Source: CAD feature listing. Evaluate the final solid. Frame: model axes, mm. Face numbers are marked on the shaded views. Round coordinates to 2 decimals unless told otherwise and drop trailing zeros. Write each loop counter-clockwise with the first axis right and the second up, starting at its lowest first coordinate (ties: lowest second). Pieces come first, ordered by that corner, then holes.
from build123d import *

# Parameters (mm, degrees)
SKETCH1_R           = 2.5
BOSS_EXTRUDE2_DEPTH = 6
SKETCH2_W           = 140.18
SKETCH2_H           = 28.64
CUT_EXTRUDE1_DEPTH  = 3


with BuildPart() as part:
    # Sketch1 → Boss-Extrude2 (new body)
    with BuildSketch(Plane(origin=(0, 0, 0), x_dir=(1, 0, 0), z_dir=(0, 1, 0))):
        Polygon((-85.09, 17.32), (-82.09, 20.32), (82.09, 20.32), (85.09, 17.32), (85.09, -17.32), (82.09, -20.32), (-82.09, -20.32), (-85.09, -17.32), align=None)
        with Locations(Location((-76.7, 12.7, 0), (0, 0, 270))):
            Circle(SKETCH1_R, mode=Mode.SUBTRACT)
        with Locations(Location((-76.7, -12.7, 0), (0, 0, 270))):
            Circle(SKETCH1_R, mode=Mode.SUBTRACT)
        with Locations(Location((76.7, 12.7, 0), (0, 0, 270))):
            Circle(SKETCH1_R, mode=Mode.SUBTRACT)
        with Locations(Location((76.7, -12.7, 0), (0, 0, 270))):
            Circle(SKETCH1_R, mode=Mode.SUBTRACT)
    extrude(amount=BOSS_EXTRUDE2_DEPTH)

    # Sketch2 → Cut-Extrude1 (cut)
    with BuildSketch(Plane(origin=(0, 6, 0), x_dir=(1, 0, 0), z_dir=(0, 1, 0))):
        Rectangle(SKETCH2_W, SKETCH2_H)
    extrude(amount=-CUT_EXTRUDE1_DEPTH, mode=Mode.SUBTRACT)


solid = part.part
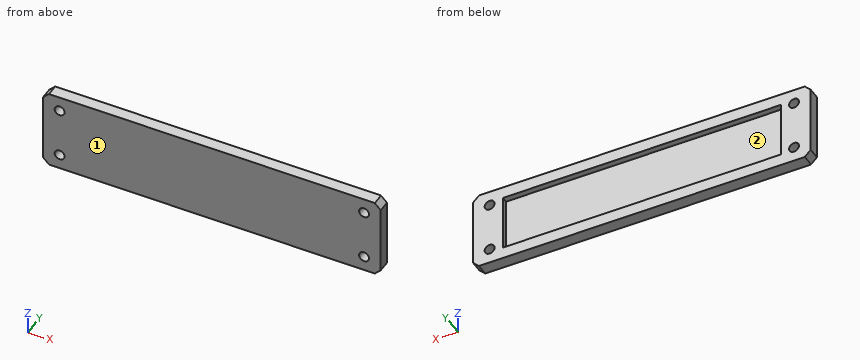
1) Contact query for a flat-ended pin moving along its axis: P1, Ø14.5, axis at x = -30, z = 2.5, coming from the +Y side. Output: stop coordinate, or through.
Taken from the geometry:
P1: stops at y = 3
2) Material intervals for line 1 (X direction, y = 3.2, z = -12.7); line 2 (X direction, y = 4.1, z = -10); line 3 (X direction, y = 2.85, z = 12.7), sorted ascending.
Taken from the geometry:
line 1: x = -85.09 to -79.2, -74.2 to -70.09, 70.09 to 74.2, 79.2 to 85.09
line 2: x = -85.09 to -70.09, 70.09 to 85.09
line 3: x = -85.09 to -79.2, -74.2 to 74.2, 79.2 to 85.09
3) Section query C-C on x = -76.7. Return the cut outline in (y, z), then the cut area to 3 significant figures.
Taken from the geometry:
outline: (0, -20.32) - (6, -20.32) - (6, -15.2) - (0, -15.2) - close; (0, -10.2) - (6, -10.2) - (6, 10.2) - (0, 10.2) - close; (0, 15.2) - (6, 15.2) - (6, 20.32) - (0, 20.32) - close
area: 184 mm2
4) Section query B-B on y = 4.75. Return the cut outline in (x, z), then the cut area to 3 significant figures.
Taken from the geometry:
outline: (-85.09, -17.32) - (-82.09, -20.32) - (82.09, -20.32) - (85.09, -17.32) - (85.09, 17.32) - (82.09, 20.32) - (-82.09, 20.32) - (-85.09, 17.32) - close; hole circle Ø5 at (-76.7, -12.7); hole circle Ø5 at (-76.7, 12.7); hole (-70.09, -14.32) - (70.09, -14.32) - (70.09, 14.32) - (-70.09, 14.32) - close; hole circle Ø5 at (76.7, -12.7); hole circle Ø5 at (76.7, 12.7)
area: 2,800 mm2
5) Section query D-D on z = 6.5. Return the cut outline in (x, y), then the cut area to 3 significant figures.
Taken from the geometry:
outline: (-85.09, 0) - (85.09, 0) - (85.09, 6) - (70.09, 6) - (70.09, 3) - (-70.09, 3) - (-70.09, 6) - (-85.09, 6) - close
area: 601 mm2
6) Section query A-A on z = 12.7. Return the cut outline in (x, y).
Taken from the geometry:
outline: (-85.09, 0) - (-79.2, 0) - (-79.2, 6) - (-85.09, 6) - close; (-74.2, 0) - (74.2, 0) - (74.2, 6) - (70.09, 6) - (70.09, 3) - (-70.09, 3) - (-70.09, 6) - (-74.2, 6) - close; (79.2, 0) - (85.09, 0) - (85.09, 6) - (79.2, 6) - close
7) Pull-direction query (X, two-part tool) for the marked faces 1 and 2; classes: released by +X, released by -X, zero draft, split by the parting line, or undercut.
Taken from the geometry:
face 1: zero draft
face 2: undercut
